from build123d import *

# Parameters (mm, degrees)
BOSS_EXTRUDE1_DEPTH = 3.175
SKETCH2_R           = 9.525
CUT_EXTRUDE1_DEPTH  = 4.175
FILLET1_R           = 1.27


with BuildPart() as part:
    # Sketch1 → Boss-Extrude1 (new body)
    with BuildSketch(Plane.XY):
        Polygon((-76.2, 12.7), (76.2, 12.7), (76.2, 22.86), (86.36, 22.86), (96.52, 2.381865319), (96.52, -10.318134681), (83.82, -20.478134681), (76.2, -20.478134681), (76.2, -12.7), (-76.2, -12.7), align=None)
    extrude(amount=BOSS_EXTRUDE1_DEPTH)

    # Sketch2 → Cut-Extrude1 (cut, through all)
    with BuildSketch(Plane.XY.offset(3.175)):
        with Locations((-63.5, 0)):
            Circle(SKETCH2_R)
        Circle(SKETCH2_R)
    extrude(amount=-CUT_EXTRUDE1_DEPTH, mode=Mode.SUBTRACT)

    # Fillet1
    fillet1_edges = [part.edges().sort_by_distance(p)[0] for p in [
        (96.52, -3.968134681, 0),
        (90.17, -15.398134681, 0),
        (80.01, -20.478134681, 0),
        (76.2, -16.58906734, 0),
        (0, -12.7, 0),
        (-76.2, 0, 0),
        (0, 12.7, 0),
        (76.2, 17.78, 3.175),
        (76.2, 17.78, 0),
        (81.28, 22.86, 0),
        (91.44, 12.62093266, 0),
        (0, 12.7, 3.175),
        (96.52, 2.381865319, 1.5875),
        (96.52, -10.318134681, 1.5875),
        (83.82, -20.478134681, 1.5875),
        (76.2, -20.478134681, 1.5875),
        (76.2, -12.7, 1.5875),
        (-76.2, -12.7, 1.5875),
        (-76.2, 12.7, 1.5875),
        (76.2, 12.7, 1.5875),
        (-76.2, 0, 3.175),
        (0, -12.7, 3.175),
        (76.2, -16.58906734, 3.175),
        (80.01, -20.478134681, 3.175),
        (90.17, -15.398134681, 3.175),
        (96.52, -3.968134681, 3.175),
        (91.44, 12.62093266, 3.175),
        (81.28, 22.86, 3.175),
    ]]
    fillet(fillet1_edges, radius=FILLET1_R)


solid = part.part
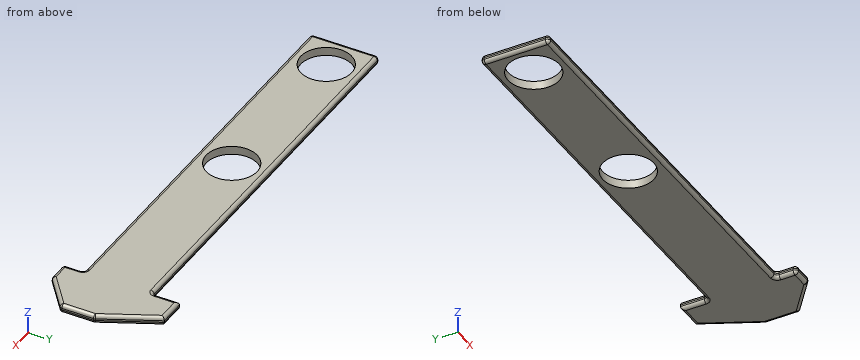
Check sheet for the modelled part. Datum: model origin and axes. Units: mm. Give positions to 0.01 mm unless a question says otherwise; leave off trailing zeros. Write each loop counter-clockwise with the first axis right and the second up, starting at its lowest first coordinate (ties: lowest second). Pieces come first, ordered by that corner, then holes. Notation, with made-up numbers: M 40.5,64 L 55.5,64 A12 ccw 55.5,69 Z; hole C 88.5,75 d11. An arc over 180 degrees is marked long. Use one line per item in the form item = value.
(1) Depth check by flat-ended pin: P1, Ø0.5, axis at x = -20, z = 1.5, coming from the +Y side; P2, Ø0.5, axis at x = -1.5, z = 1.5, coming from the -Y side. Enter the tip coordinate at first touch or a pass-through.
Answer block:
P1 = 12.7
P2 = -12.7
(2) Material ranges on line 1 along Y through (x, z) = (0, 1.6) (3 decimals); line 2 along X through (y, z) = (1.5, 2.85); line 3 along Y through (x, z) = (-8, 2.9), recorded low to high.
Answer block:
line_1 = -12.7 to -9.525, 9.525 to 12.7
line_2 = -75.78 to -72.91, -54.09 to -9.41, 9.41 to 96.1
line_3 = -12.22 to -5.17, 5.17 to 12.22
(3) Section check A-A on y = 0. Record the boundary of the cut face in (x, z) (3 decimals), plus the area to 3 significant figures.
Answer block:
outline = M -76.2,1.27 A1.27 ccw -74.93,0 L -73.025,0 L -73.025,3.175 L -74.93,3.175 A1.27 ccw -76.2,1.905 Z; M -53.975,0 L -9.525,0 L -9.525,3.175 L -53.975,3.175 Z; M 9.525,0 L 95.25,0 A1.27 ccw 96.52,1.27 L 96.52,1.905 A1.27 ccw 95.25,3.175 L 9.525,3.175 Z
area = 426 mm2
(4) Section check B-B on x = 0. Record the boundary of the cut face in (y, z) (3 decimals).
Answer block:
outline = M -12.7,1.27 A1.27 ccw -11.43,0 L -9.525,0 L -9.525,3.175 L -11.43,3.175 A1.27 ccw -12.7,1.905 Z; M 9.525,0 L 11.43,0 A1.27 ccw 12.7,1.27 L 12.7,1.905 A1.27 ccw 11.43,3.175 L 9.525,3.175 Z
(5) Section check C-C on x = 41. Record the boundary of the cut face in (y, z) (3 decimals).
Answer block:
outline = M -12.7,1.27 A1.27 ccw -11.43,0 L 11.43,0 A1.27 ccw 12.7,1.27 L 12.7,1.905 A1.27 ccw 11.43,3.175 L -11.43,3.175 A1.27 ccw -12.7,1.905 Z
